from build123d import *

# Parameters (mm, degrees)
F0_W     = 76.2
F0_H     = 50.8
F1_DEPTH = 9.525
F2_W     = 25.4
F2_H     = 12.7
F2_H_2   = 25.4
F3_DEPTH = 19.05
F4_DEPTH = 9.525


with BuildPart() as f1:
    # F0 (on Top) → F1 (new body)
    with BuildSketch(Plane.XY):
        Rectangle(F0_W, F0_H)
    extrude(amount=F1_DEPTH)

    # F2 (on face) → F3 (join)
    with BuildSketch(Plane.XY.offset(9.525)):
        with Locations((-25.4, 19.05)):
            Rectangle(F2_W, F2_H)
        with Locations((-25.4, 0)):
            Rectangle(F2_W, F2_H_2)
        with Locations((-25.4, -19.05)):
            Rectangle(F2_W, F2_H)
    extrude(amount=F3_DEPTH)

    # F2 (on face) → F4 (join)
    with BuildSketch(Plane.XY.offset(9.525)):
        with Locations((-25.4, 19.05)):
            Rectangle(F2_W, F2_H)
        with Locations((0, 19.05)):
            Rectangle(F2_W, F2_H)
        with Locations((-25.4, 0)):
            Rectangle(F2_W, F2_H_2)
        with Locations((-25.4, -19.05)):
            Rectangle(F2_W, F2_H)
        with Locations((0, -19.05)):
            Rectangle(F2_W, F2_H)
    extrude(amount=F4_DEPTH)


solid = f1.part
Design review of the part built by this model. Coordinates are the model's own, in mm. A direction names the side the tool comes from. Coordinates: 2 decimals unless noted, no trailing zeros. Write each loop counter-clockwise with the first axis right and the second up, starting at its lowest first coordinate (ties: lowest second). Pieces come first, ordered by that corner, then holes. Notation, with made-up numbers: (-2.5, 58) -> (56.5, 58) arc R33 ccw to (56.5, 95) -> close; hole circle Ø11 at (-2, 9.25). An arc over 180 degrees is marked (long way). Write each question's results on one line, items separated by ' | '. Start each with the question number.
(1) Take a section at A-A on z = 13.75. Write out the cut boundary in (x, y).
(2) Clearance check with flat-ended pins moving along their axes: P1, Ø3, axis at x = -5, z = 22.5, coming from the +Y side; P2, Ø5, axis at y = 14.5, z = 18.5, coming from the +X side; P3, Ø14, axis at x = -3, y = -18, coming from the +Z side. State where each tip first meets the part, or that it passes through.
(3) The part is to be moulded in two halves that separate along Y. For faces 1 (the face through (-9, 25.4, 11)), 2 (the face through (0, -12.7, 14)), 3 (the face through (-26, 0, 28.575)), 4 (the face through (-9, -25.4, 11)), say which applies: pulls with the +Y half, pulls with the -Y half, needs draft (parallel to the pull), parting line crosses it, or undercut.
(4) Take a section at B-B on x = -11. Write out the cut boundary in (y, z) (3 decimals), and give its area (3 significant figures).
(5) Take a section at D-D on z = 20.25. Write out the cut boundary in (x, y), and give its area (3 significant figures).
(6) Tool access review of faces 5 (the face through (-1, 0, 0)), 6 (the face through (12.7, -19, 14)), 7 (the face through (0, 12.7, 14)): name each direction out of +Z, -Z, +X, -X, +Y, -Y from which nothing blocks a thin tool from reaching the whole face with its end or side.
(7) Take a section at C-C on y = -1. Write out the cut boundary in (x, z) (3 decimals).
(8) For line 1 along Y through (x, z) = (11.5, 16.5); line 2 along Z through (x, y) = (2, -1) (3 decimals); line 3 along Z through (x, y) = (12, 18.5), list the stretches that pass through material, from the lowest coordinate up. Write a range as from..to.
Results found:
1) outline: (-38.1, -25.4) -> (12.7, -25.4) -> (12.7, -12.7) -> (-12.7, -12.7) -> (-12.7, 12.7) -> (12.7, 12.7) -> (12.7, 25.4) -> (-38.1, 25.4) -> close
2) P1: passes through | P2: stops at x = 12.7 | P3: stops at z = 19.05
3) face 1: pulls with the +Y half | face 2: undercut | face 3: needs draft | face 4: pulls with the -Y half
4) outline: (-25.4, 0) -> (25.4, 0) -> (25.4, 19.05) -> (12.7, 19.05) -> (12.7, 9.525) -> (-12.7, 9.525) -> (-12.7, 19.05) -> (-25.4, 19.05) -> close | area: 726 mm2
5) outline: (-38.1, -25.4) -> (-12.7, -25.4) -> (-12.7, 25.4) -> (-38.1, 25.4) -> close | area: 1,290 mm2
6) face 5: -Z, +X, -X, +Y, -Y | face 6: +Z, +X, +Y, -Y | face 7: +Z, +X
7) outline: (-38.1, 0) -> (38.1, 0) -> (38.1, 9.525) -> (-12.7, 9.525) -> (-12.7, 28.575) -> (-38.1, 28.575) -> close
8) line 1: y = -25.4..-12.7, 12.7..25.4 | line 2: z = 0..9.525 | line 3: z = 0..19.05
